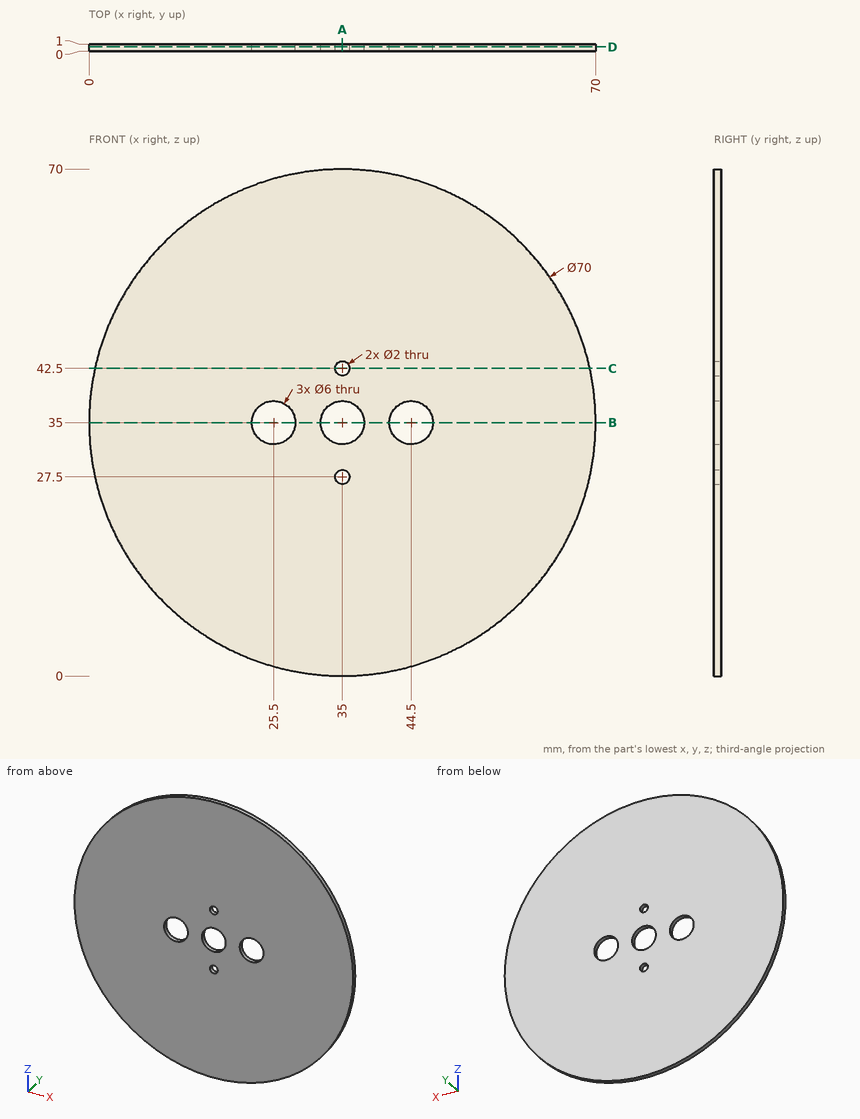
Verification items for this drawing (mm, ordinates from the low corner). Give positions to 0.01 mm unless a question says otherwise; leave off trailing zeros. Loops run counter-clockwise (first coordinate to the right, second up) from the corner with the lowest first, then second, coordinate; pieces in that order, holes last. Notation, with made-up numbers: M -39.75,47.25 L -23.75,47.25 A16 cw -23.75,66.25 Z; hole C 31.5,82 d10. An arc over 180 degrees is marked long. Write item = value, one per line.
(1) Sectioned sample at B-B, the plane z = 35. Record the cut outline in (x, y), plus the area to 3 significant figures.
Answer below:
outline = M 0,0 L 22.5,0 L 22.5,1 L 0,1 Z; M 28.5,0 L 32,0 L 32,1 L 28.5,1 Z; M 38,0 L 41.5,0 L 41.5,1 L 38,1 Z; M 47.5,0 L 70,0 L 70,1 L 47.5,1 Z
area = 52.0 mm2
(2) Gauge pin test, flat end, axial feed: pin 1 Ø5 at (x, z) = (35, 35) entering from -Y. Record the tip position at first contact, or that the pin passes through.
Answer below:
pin_1 = through
(3) Material ranges on line 1 (Z direction, x = 35, y = 0.8); line 2 (X direction, y = 0.35, z = 35.5); line 3 (X direction, y = 0.4, z = 34), recorded low to high. Write a range as [from, to].
Answer below:
line_1 = [0, 26.5], [28.5, 32], [38, 41.5], [43.5, 70]
line_2 = [0, 22.54], [28.46, 32.04], [37.96, 41.54], [47.46, 70]
line_3 = [0.01, 22.67], [28.33, 32.17], [37.83, 41.67], [47.33, 69.99]
(4) Sectioned sample at A-A, the plane x = 35. Record the cut outline in (y, z).
Answer below:
outline = M 0,0 L 1,0 L 1,26.5 L 0,26.5 Z; M 0,28.5 L 1,28.5 L 1,32 L 0,32 Z; M 0,38 L 1,38 L 1,41.5 L 0,41.5 Z; M 0,43.5 L 1,43.5 L 1,70 L 0,70 Z
(5) Sectioned sample at C-C, the plane z = 42.5. Record the cut outline in (x, y), plus the area to 3 significant figures.
Answer below:
outline = M 0.81,0 L 34,0 L 34,1 L 0.81,1 Z; M 36,0 L 69.19,0 L 69.19,1 L 36,1 Z
area = 66.4 mm2
(6) Sectioned sample at D-D, the plane y = 0.6. Record the cut outline in (x, z).
Answer below:
outline = C 35,35 d70; hole C 25.5,35 d6; hole C 35,35 d6; hole C 35,27.5 d2; hole C 35,42.5 d2; hole C 44.5,35 d6
